Check sheet for the drawn part. Datum: minimum x, y, z corner. Units: mm. A direction names the side the tool comes from. Round coordinates to 2 decimals unless told otherwise and drop trailing zeros. Write each loop counter-clockwise with the first axis right and the second up, starting at its lowest first coordinate (ties: lowest second). Pieces come first, ordered by that corner, then holes. Notation, with made-up numbers: (67.5, 41.5) - (94.5, 41.5) arc R26 cw to (94.5, 61.5) - close; hole circle Ø5 at (70, -3). An arc over 180 degrees is marked (long way). Answer as a JSON object with one key per item and string values. Group by question number.
Item 1: Gauge pin test, flat end, axial feed: P1, Ø2, axis at x = 1.5, y = 4, coming from the -Z side. Record the tip position at first contact, or that the pin passes through.
Item 2: Set-up check for the marked faces 1 and 2: record each of +Z, -Z, +X, -X, +Y, -Y from which the full face is reachable in a straight line by a thin tool's end or side.
Item 3: Sectioned sample at B-B on y = 2.25. Record the boundary of the cut face in (x, z).
Item 4: Release check for a two-part mould opening along X. For the marked faces 3, 4 and 5 record: pulls with the +X half, pulls with the -X half, needs draft (parallel to the pull), parting line crosses it, or undercut.
Item 5: Thickness scan on line 1 (Y direction, x = 2.9, z = 3.25); line 2 (Y direction, x = 2.9, z = 1); line 3 (X direction, y = 21.5, z = 3.25). Record the ranges inside material, lowest first.
Item 6: Sectioned sample at A-A on y = 14. Record the boundary of the cut face in (x, z).
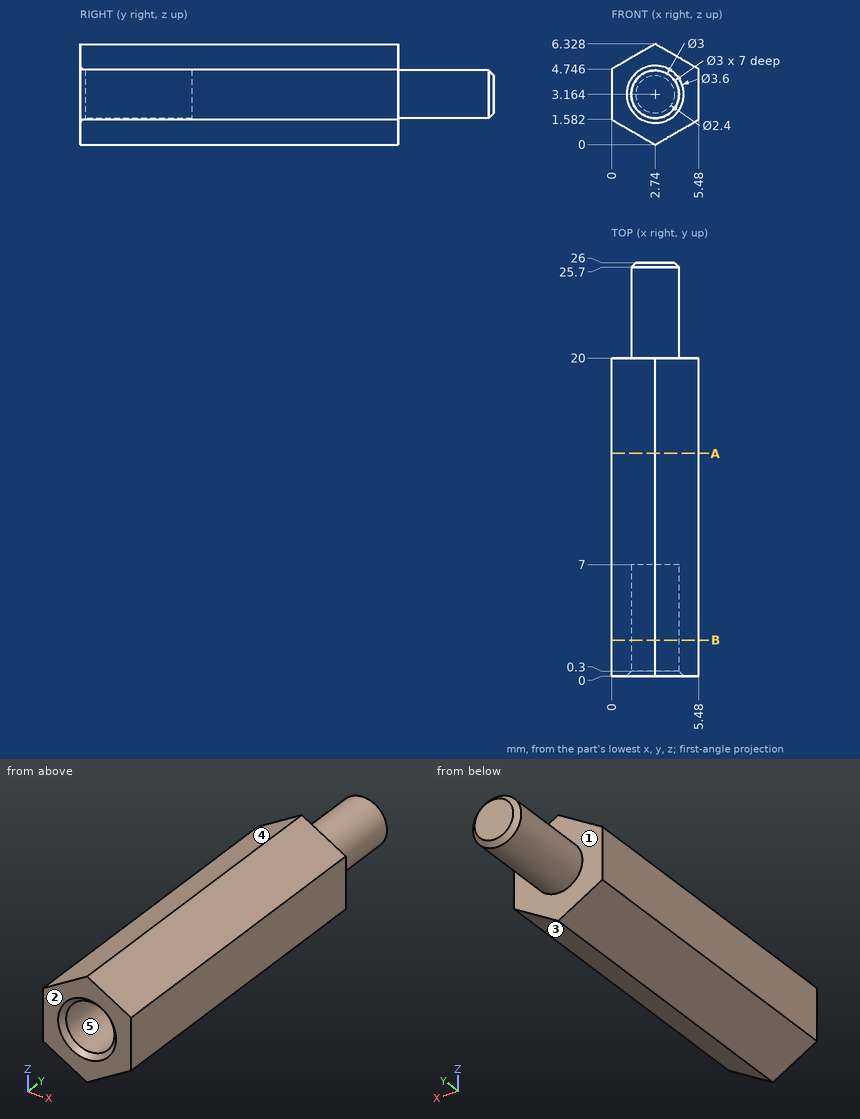
Completed:
{
 "1": {"P1": "z = 0.14"},
 "2": {"face 1": "+Y", "face 2": "+Z, -Z, +X, -X, -Y"},
 "3": {"outline": "(0, 1.58) - (2.74, 0) - (5.48, 1.58) - (5.48, 4.75) - (2.74, 6.33) - (0, 4.75) - close; hole circle Ø3 at (2.74, 3.16)"},
 "4": {"face 3": "pulls with the +X half", "face 4": "pulls with the -X half", "face 5": "undercut"},
 "5": {"line 1": "7 to 26", "line 2": "0 to 20", "line 3": "1.24 to 4.24"},
 "6": {"outline": "(0, 1.58) - (2.74, 0) - (5.48, 1.58) - (5.48, 4.75) - (2.74, 6.33) - (0, 4.75) - close"}
}
